```python
from build123d import *

# Parameters (mm, degrees)
F0_W     = 40
F0_H     = 15
F0_R     = 1
F0_R_2   = 1.5
F1_DEPTH = 6
F2_SIZE  = 2


with BuildPart() as f1:
    # F0 (on Front) → F1 (new body)
    with BuildSketch(Plane.XZ):
        Rectangle(F0_W, F0_H)
        with Locations((14.75, -3.2)):
            Circle(F0_R, mode=Mode.SUBTRACT)
        with Locations((-10, 0)):
            Circle(F0_R_2, mode=Mode.SUBTRACT)
        with Locations((10, 0)):
            Circle(F0_R_2, mode=Mode.SUBTRACT)
        with Locations((14.75, 3.2)):
            Circle(F0_R, mode=Mode.SUBTRACT)
    extrude(amount=F1_DEPTH)

    # F2
    f2_edges = [f1.edges().sort_by_distance(p)[0] for p in [
        (-11.5, -6, 0),
        (8.5, -6, 0),
    ]]
    chamfer(f2_edges, length=F2_SIZE)


solid = f1.part
```
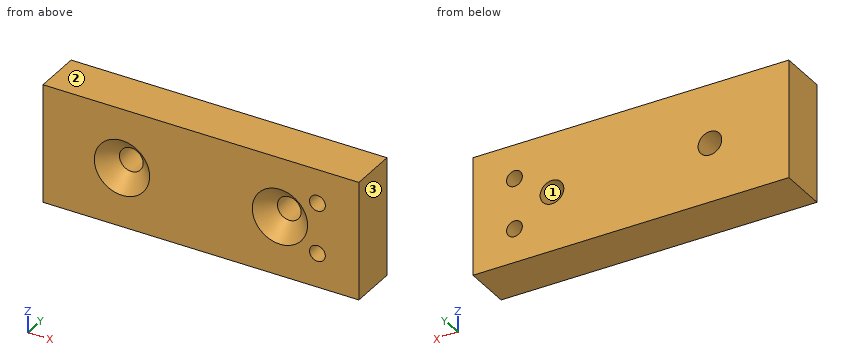
Verification items for the finished model (mm, model axes). Face numbers are marked on the shaded views. Give positions to 0.01 mm unless a question says otherwise; leave off trailing zeros. Loops run counter-clockwise (first coordinate to the right, second up) from the corner with the lowest first, then second, coordinate; pieces in that order, holes last.
1. Section check B-B, the plane y = -1.8. Enter the section's corners in (x, z), then the cut area to 3 significant figures.
2. Thickness scan on line 1 (Z direction, x = 14.75, y = -3); line 2 (Z direction, x = 10, y = -1.65); line 3 (X direction, y = -2.95, z = 0.5). Record the ranges inside material, lowest first.
3. Section check A-A, the plane x = 10. Enter the section's corners in (y, z).
4. Section check D-D, the plane x = 14.75. Enter the section's corners in (y, z), then the cut area to 3 significant figures.
5. Mould release check, pull along X, two halves, no side actions. Record for the marked faces 1, 2 and 3: released by +X, released by -X, zero draft, split by the parting line, or undercut.
6. Section check C-C, the plane z = 0. Enter the section's corners in (x, y), then the cut area to 3 significant figures.
7. Go/stop test with flat-tipped pins: pin 1 Ø3 at (x, z) = (15, -2) entering from +Y; pin 2 Ø3.5 at (x, z) = (10, 0) entering from -Y. Record where each tip stops, or that it passes through.
Geometry says:
1. outline: (-20, -7.5) - (20, -7.5) - (20, 7.5) - (-20, 7.5) - close; hole circle Ø3 at (-10, 0); hole circle Ø3 at (10, 0); hole circle Ø2 at (14.75, -3.2); hole circle Ø2 at (14.75, 3.2)
1. area: 580 mm2
2. line 1: z = -7.5 to -4.2, -2.2 to 2.2, 4.2 to 7.5
2. line 2: z = -7.5 to -1.5, 1.5 to 7.5
2. line 3: x = -20 to -11.41, -8.59 to 8.59, 11.41 to 20
3. outline: (-6, -7.5) - (0, -7.5) - (0, -1.5) - (-4, -1.5) - (-6, -3.5) - close; (-6, 3.5) - (-4, 1.5) - (0, 1.5) - (0, 7.5) - (-6, 7.5) - close
4. outline: (-6, -7.5) - (0, -7.5) - (0, -4.2) - (-6, -4.2) - close; (-6, -2.2) - (0, -2.2) - (0, 2.2) - (-6, 2.2) - close; (-6, 4.2) - (0, 4.2) - (0, 7.5) - (-6, 7.5) - close
4. area: 66.0 mm2
5. face 1: undercut
5. face 2: zero draft
5. face 3: released by +X
6. outline: (-20, -6) - (-13.5, -6) - (-11.5, -4) - (-11.5, 0) - (-20, 0) - close; (-8.5, -4) - (-6.5, -6) - (6.5, -6) - (8.5, -4) - (8.5, 0) - (-8.5, 0) - close; (11.5, -4) - (13.5, -6) - (20, -6) - (20, 0) - (11.5, 0) - close
6. area: 196 mm2
7. pin 1: stops at y = 0
7. pin 2: stops at y = -4.25
